```python
from build123d import *

# Parameters (mm, degrees)
ESQUISSE1_W             = 84
ESQUISSE1_H             = 115
BOSS_EXTRU_1_DEPTH      = 58
ESQUISSE2_W             = 110
ESQUISSE2_H             = 48
ENL_V_MAT_EXTRU_1_DEPTH = 4


with BuildPart() as part:
    # Esquisse1 → Boss.-Extru.1 (new body)
    with BuildSketch(Plane(origin=(0, 0, 0), x_dir=(1, 0, 0), z_dir=(0, 1, 0))):
        Rectangle(ESQUISSE1_W, ESQUISSE1_H)
    extrude(amount=BOSS_EXTRU_1_DEPTH)

    # Esquisse2 → Enlèv. mat.-Extru.1 (cut)
    with BuildSketch(Plane.ZY.offset(42)):
        with Locations((2.5, 29)):
            Rectangle(ESQUISSE2_W, ESQUISSE2_H)
    enl_v_mat_extru_1 = extrude(amount=-ENL_V_MAT_EXTRU_1_DEPTH, mode=Mode.SUBTRACT)

    # Symétrie1: Enlèv. mat.-Extru.1 across plane
    add(enl_v_mat_extru_1.mirror(Plane(origin=(0, 0, 0), x_dir=(0, 0, 1), z_dir=(1, 0, 0))), mode=Mode.SUBTRACT)


solid = part.part
```
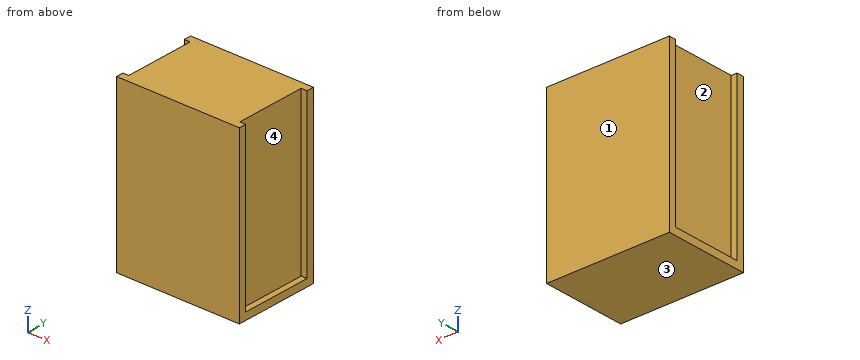
Build history of the part. All positions in model axes, mm. Face numbers are marked on the shaded views. Coordinates: 2 decimals unless noted, no trailing zeros. Order: outer loops, then holes, each group sorted by start corner. A loop starts at its lowest first (then second) coordinate and runs counter-clockwise, first axis right, second up. Notation, with made-up numbers: M 25,34 L 82,34 A23 cw 82,63 Z; hole C 83,3 d10. An arc over 180 degrees is marked long. One line per question, with ' | ' between items. Start each with the question number.
1. Flat gauge pins, fed straight in: P1, Ø2, axis at y = 16, z = 10, coming from the -X side; P2, Ø4.5, axis at x = 40.5, y = 26, coming from the +Z side; P3, Ø10, axis at y = 15, z = 22.5, coming from the +X side. Where does each tip first touch, or does it go through?
2. Cut at B-B (z = 22). Write the cut outline in (x, y), plus the area to 3 significant figures.
3. Mould opens along Y. For the marked faces 1, 2, 3 and 4 say: +Y half, -Y half, draft (parallel to the pull), parting line (faces both ways), or undercut.
4. Wall check: line 1 along X through (y, z) = (41.5, 16.5). Give the ranges that are in metal, low to high. Write a range as [from, to].
5. Cut at A-A (y = 30.5). Write the cut outline in (x, z), plus the area to 3 significant figures.
The answers:
1) P1: stops at x = -38 | P2: stops at z = -52.5 | P3: stops at x = 38
2) outline: M -42,0 L 42,0 L 42,5 L 38,5 L 38,53 L 42,53 L 42,58 L -42,58 L -42,53 L -38,53 L -38,5 L -42,5 Z | area: 4,490 mm2
3) face 1: +Y half | face 2: undercut | face 3: draft | face 4: undercut
4) line 1: x = [-38, 38]
5) outline: M -42,-57.5 L 42,-57.5 L 42,-52.5 L 38,-52.5 L 38,57.5 L -38,57.5 L -38,-52.5 L -42,-52.5 Z | area: 8,780 mm2
